```python
from build123d import *

# Parameters (mm, degrees)
ESQUISSE1_W             = 116
ESQUISSE1_H             = 83
BOSS_EXTRU_1_DEPTH      = 4
CONG_1_R                = 5
ESQUISSE2_R             = 2
ESQUISSE2_R_2           = 11.5
ENL_V_MAT_EXTRU_1_DEPTH = 4
ESQUISSE3_R             = 3
ENL_V_MAT_EXTRU_2_DEPTH = 2.5
ENL_V_START             = -4
ENL_V_MAT_EXTRU_3_DEPTH = 2.2


with BuildPart() as part:
    # Esquisse1 → Boss.-Extru.1 (new body)
    with BuildSketch(Plane.XY):
        with Locations((0.978902954, 8.301687764)):
            Rectangle(ESQUISSE1_W, ESQUISSE1_H)
    extrude(amount=BOSS_EXTRU_1_DEPTH)

    # Congé1
    cong_1_edges = [part.edges().sort_by_distance(p)[0] for p in [
        (-57.021097046, 49.801687764, 2),
        (58.978902954, 49.801687764, 2),
        (58.978902954, -33.198312236, 2),
        (-57.021097046, -33.198312236, 2),
    ]]
    fillet(cong_1_edges, radius=CONG_1_R)

    # Esquisse2 → Enlèv. mat.-Extru.1 (cut)
    with BuildSketch(Plane.XY.offset(4)):
        with Locations((-42.021097046, -28.198312236)):
            Circle(ESQUISSE2_R)
        with Locations((-52.021097046, 44.801687764)):
            Circle(ESQUISSE2_R)
        with Locations((-21.021097046, 44.801687764)):
            Circle(ESQUISSE2_R)
        with Locations((-36.521097046, 29.301687764)):
            Circle(ESQUISSE2_R_2)
        with Locations((-21.021097046, 13.801687764)):
            Circle(ESQUISSE2_R)
        with Locations((-52.021097046, 13.801687764)):
            Circle(ESQUISSE2_R)
        with Locations(Location((43.978902954, -28.198312236, 0), (0, 0, 180))):
            Circle(ESQUISSE2_R)
        with Locations(Location((38.478902954, 29.301687764, 0), (0, 0, 180))):
            Circle(ESQUISSE2_R_2)
        with Locations(Location((22.978902954, 13.801687764, 0), (0, 0, 180))):
            Circle(ESQUISSE2_R)
        with Locations(Location((22.978902954, 44.801687764, 0), (0, 0, 180))):
            Circle(ESQUISSE2_R)
        with Locations(Location((53.978902954, 44.801687764, 0), (0, 0, 180))):
            Circle(ESQUISSE2_R)
        with Locations(Location((53.978902954, 13.801687764, 0), (0, 0, 180))):
            Circle(ESQUISSE2_R)
    extrude(amount=-ENL_V_MAT_EXTRU_1_DEPTH, mode=Mode.SUBTRACT)

    # Esquisse3 → Enlèv. mat.-Extru.2 (cut)
    with BuildSketch(Plane.XY.offset(4)):
        with Locations((-52.021097046, 13.801687764)):
            Circle(ESQUISSE3_R)
        with Locations((-21.021097046, 13.801687764)):
            Circle(ESQUISSE3_R)
        with Locations((22.978902954, 13.801687764)):
            Circle(ESQUISSE3_R)
        with Locations((53.978902954, 13.801687764)):
            Circle(ESQUISSE3_R)
    extrude(amount=-ENL_V_MAT_EXTRU_2_DEPTH, mode=Mode.SUBTRACT)

    # Esquisse4 → Enlèv. mat.-Extru.3 (cut)
    with BuildSketch(Plane.XY.offset(4).offset(ENL_V_START)):
        Polygon((-43.753147854, -25.198312236), (-45.485198662, -28.198312236), (-43.753147854, -31.198312236), (-40.289046239, -31.198312236), (-38.556995431, -28.198312236), (-40.289046239, -25.198312236), align=None)
        Polygon((42.246852146, -25.198312236), (40.514801338, -28.198312236), (42.246852146, -31.198312236), (45.710953761, -31.198312236), (47.443004569, -28.198312236), (45.710953761, -25.198312236), align=None)
    extrude(amount=ENL_V_MAT_EXTRU_3_DEPTH, mode=Mode.SUBTRACT)


solid = part.part
```
The model under review builds one solid part; all positions refer to its coordinate system, in mm. A direction names the side the tool comes from. Round coordinates to 2 decimals unless told otherwise and drop trailing zeros. Order: outer loops, then holes, each group sorted by start corner. A loop starts at its lowest first (then second) coordinate and runs counter-clockwise, first axis right, second up. Notation, with made-up numbers: (0, 51.25) -> (34, 51.25) arc R12 cw to (34, 63.25) -> close; hole circle Ø7 at (1.25, 85.5). An arc over 180 degrees is marked (long way). One line per item, written item: value. Start each with the question number.
Q1. Take a section at C-C (z = 3.3). Count the separate pieces of the cut face and the enclosed holes in it, and give its area (3 significant figures).
Q2. Machinability: for faces 4 (the face through (-39.41, -26.72, 1.08)), 5 (the face through (53.329, 10.873, 2.768)), 6 (the face through (0, 9, 0)), which of the approach directions +Z, -Z, +X, -X, +Y, -Y give a long, thin tool a straight path to every point of the face, cutting with its end or side? Answer none if there is none.
Q3. Clearance check with a flat-ended pin moving along its axis: pin 1 Ø3 at (x, y) = (-21.5, 13.5) entering from +Z. State where the tip first meets the part, or that it passes through.
Q4. Take a section at B-B (y = 39.5). Write out the cut boundary in (x, z).
Q5. Mouldability with a two-part tool opening along Y and no side actions: class faces 1 (the face through (-44.63, -29.68, 1.08)), 2 (the face through (-57.021, 8, 2)), 3 (the face through (0, 49.802, 2)) as released by +Y, released by -Y, zero draft, split by the parting line, or undercut.
Q6. Take a section at A-A (x = -31). Write out the cut boundary in (y, z).
Q7. Wall thickness on line 1 (Y direction, x = -52, z = 0.55); line 2 (X direction, y = -28, z = 2.9); line 3 (Y direction, x = -36, z = 2.7): over which ranges is each line inside the solid? List them lowest first.
Reported:
1. separate pieces: 1
1. enclosed holes: 12
1. area: 8,590 mm2
2. face 4: -Z
2. face 5: +Z
2. face 6: -Z, +X, -X, +Y, -Y
3. pin 1: stops at z = 1.5
4. outline: (-57.02, 0) -> (-41.84, 0) -> (-41.84, 4) -> (-57.02, 4) -> close; (-31.21, 0) -> (33.16, 0) -> (33.16, 4) -> (-31.21, 4) -> close; (43.79, 0) -> (58.98, 0) -> (58.98, 4) -> (43.79, 4) -> close
5. face 1: undercut
5. face 2: zero draft
5. face 3: released by +Y
6. outline: (-33.2, 0) -> (19.21, 0) -> (19.21, 4) -> (-33.2, 4) -> close; (39.39, 0) -> (49.8, 0) -> (49.8, 4) -> (39.39, 4) -> close
7. line 1: y = -33.2 to 11.8, 15.8 to 42.8, 46.8 to 49.8
7. line 2: x = -57.02 to -44.01, -40.03 to 41.99, 45.97 to 58.98
7. line 3: y = -33.2 to 17.81, 40.79 to 49.8
